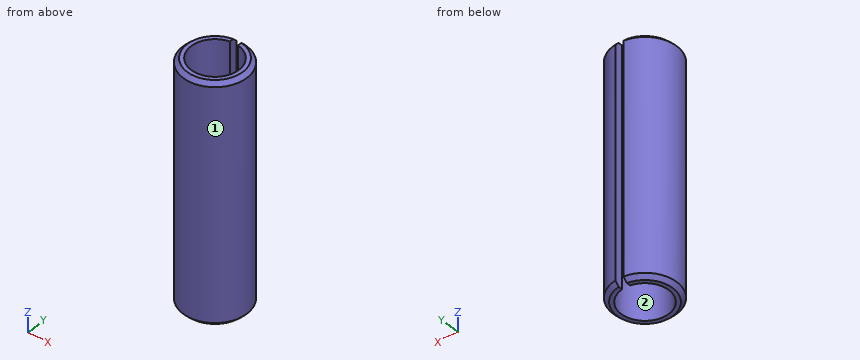
```python
from build123d import *

# Parameters (mm, degrees)
EXTRUSION1_DEPTH      = 15
EXTRUSION1_DEPTH_BACK = 15
CHANFREIN1_SIZE       = 0.5


with BuildPart() as part:
    # Esquisse1 → Extrusion1 (new body, two sides)
    with BuildSketch(Plane.XY) as extrusion1_sk:
        with BuildLine():
            Line((0.5, 3.968626967), (0.5, 2.958039892))
            ThreePointArc((0.5, 2.958039892), (0, -3), (-0.5, 2.958039892))
            Line((-0.5, 2.958039892), (-0.5, 3.968626967))
            ThreePointArc((-0.5, 3.968626967), (0, -4), (0.5, 3.968626967))
        make_face()
    extrude(amount=EXTRUSION1_DEPTH)
    extrude(extrusion1_sk.sketch, amount=-EXTRUSION1_DEPTH_BACK)

    # Chanfrein1
    chanfrein1_edges = [part.edges().sort_by_distance(p)[0] for p in [
        (0, -4, -15),
        (0, -4, 15),
    ]]
    chamfer(chanfrein1_edges, length=CHANFREIN1_SIZE)


solid = part.part
```
Read the model definition and answer for the solid it produces. Units are mm, in the model's axes. Face numbers are marked on the shaded views. Give positions to 0.01 mm unless a question says otherwise; leave off trailing zeros. Order: outer loops, then holes, each group sorted by start corner. A loop starts at its lowest first (then second) coordinate and runs counter-clockwise, first axis right, second up.
(1) Straight lines are drawn through the part: L1, parallel to X at y = 0, z = -8; L2, parallel to X at y = -1, z = -3.5; L3, parallel to Y at x = -2.75, z = 4.5. For each, find the intervals that lie inside material, in ascending order.
(2) Given pin 1 (1.5 mm diameter, centred on y = -2.5, z = 9.5, fed in from -X); pin 2 (1.5 mm diameter, centred on y = 2.5, z = -10, fed in from +X); pin 3 (0.8 mm diameter, centred on y = 3.5, z = -2.5, fed in from -X), each flat-ended and moving along its own axis, determine where each tip first touches the part or whether it passes through.
(3) Find section A-A (y = 0). Give the vertices of the cut face in (x, z).
(4) Find section C-C (z = 7). Give the vertices of the cut face in (x, y).
(5) For a pull along Y with two mould halves and no side action, classify the marked faces 1 and 2 as released by +Y, released by -Y, zero draft, split by the parting line, or undercut.
(6) Find section B-B (x = 0). Give the vertices of the cut face in (y, z), plus the area to 4 significant figures.
Result sheet:
1. L1: x = -4 to -3, 3 to 4
1. L2: x = -3.87 to -2.83, 2.83 to 3.87
1. L3: y = -2.9 to -1.2, 1.2 to 2.9
2. pin 1: stops at x = -3.6
2. pin 2: stops at x = 3.6
2. pin 3: stops at x = -2.53
3. outline: (-4, -14.5) - (-3.5, -15) - (-3, -15) - (-3, 15) - (-3.5, 15) - (-4, 14.5) - close; (3, -15) - (3.5, -15) - (4, -14.5) - (4, 14.5) - (3.5, 15) - (3, 15) - close
4. outline: (-0.5, 2.96) - (-0.5, 3.97) arc R4 ccw (long way) to (0.5, 3.97) - (0.5, 2.96) arc R3 cw (long way) to start
5. face 1: split by the parting line
5. face 2: undercut
6. outline: (-4, -14.5) - (-3.5, -15) - (-3, -15) - (-3, 15) - (-3.5, 15) - (-4, 14.5) - close
6. area: 29.75 mm2
